from build123d import *

# Parameters (mm, degrees)
F0_W     = 10.922
F0_H     = 25.4
F4_W     = 0.635
F4_H     = 3.81
F6_R     = 1.5875
F7_DEPTH = 12.7
F8_R     = 3.175
F9_DEPTH = 6.35


with BuildPart() as f1:
    # F0 (on Front) → F1 (revolve)
    with BuildSketch(Plane.XZ):
        with Locations((5.461, 0)):
            Rectangle(F0_W, F0_H)
    revolve(axis=Axis((0, 0, 0), (0, 0, -1)))

    # F2 (on face) → F3 (revolve, cut)
    with BuildSketch(Plane(origin=(0, 0, -12.7), x_dir=(1, 0, 0), z_dir=(0, 0, -1))):
        with BuildLine():
            Line((0, 10.287), (0, -10.287))
            ThreePointArc((0, -10.287), (10.287, 0), (0, 10.287))
        make_face()
    revolve(axis=Axis((0, 0, -12.7), (0, 1, 0)), mode=Mode.SUBTRACT)

    # F4 (on Front) → F5 (revolve)
    with BuildSketch(Plane.XZ):
        with Locations((10.6045, -14.605)):
            Rectangle(F4_W, F4_H)
    revolve(axis=Axis((0, 0, -6.3285445794), (0, 0, -1)))

    # F6 (on Right) → F7 (cut, symmetric)
    with BuildSketch(Plane.YZ):
        with Locations((0, -14.478)):
            Circle(F6_R)
    extrude(amount=F7_DEPTH, both=True, mode=Mode.SUBTRACT)

    # F8 (on face) → F9 (join)
    with BuildSketch(Plane.XY.offset(12.7)):
        Circle(F8_R)
    extrude(amount=F9_DEPTH)


solid = f1.part
Build history of the part. All positions in model axes, mm. A direction names the side the tool comes from. Coordinates: 2 decimals unless noted, no trailing zeros. Order: outer loops, then holes, each group sorted by start corner. A loop starts at its lowest first (then second) coordinate and runs counter-clockwise, first axis right, second up. Notation, with made-up numbers: M 34,67 L 89,67 A24 cw 89,82 Z; hole C 23.25,87.5 d11. An arc over 180 degrees is marked long. One line per question, with ' | ' between items. Start each with the question number.
Q1. Saw through at B-B (x = -0.5). List the corners of the cut face in (y, z).
Q2. Saw through at C-C (y = -6.75). List the corners of the cut face in (x, z), then the cut area to 3 significant figures.
Q3. Saw through at D-D (z = -2). List the corners of the cut face in (x, y).
Q4. Saw through at A-A (y = 0). Count the separate pieces of the cut face and the enclosed holes in it, then the cut area to 3 significant figures.
Q5. Flat gauge pins, fed straight in: pin 1 Ø3 at (x, z) = (-3, 9.5) entering from +Y; pin 2 Ø2 at (y, z) = (-2.5, -1.5) entering from -X; pin 3 Ø2 at (x, z) = (1, 4) entering from -Y; pin 4 Ø1.5 at (x, y) = (-0.5, -6.5) entering from -Z. Where does each tip first touch, or does it go through?
Q6. Probe L1, parallel to Z at x = 10.45, y = 0; L2, parallel to Y at x = 0, z = -14.1; L3, parallel to Z at x = -9.5, y = 4.75. List the from-to ranges inside material, lowest first. Write a range as from..to.
Q7. Two-plate mould, pull along Y, no slides. Class faces 3 (the face through (0, 0, 19.05)), 4 (the face through (9.81, -3.09, -14.58)), 5 (the face through (10.09, 4.18, -1.7)): +Y half, -Y half, draft (parallel to the pull), parting line (faces both ways), or undercut.
Q8. 3-axis set-ups, long thin cutter, end or side, ignore diameter. For faces 1 (the face through (-0.69, -3.1, 15.83)), 2 (the face through (10.548, 1.466, -15.086)): which of +Z, -Z, +X, -X, +Y, -Y reach the whole face in a straight line?
Check values:
1) outline: M -10.91,-16.51 L -10.27,-16.51 L -10.27,-12.7 A10.27 cw 10.27,-12.7 L 10.27,-16.51 L 10.91,-16.51 L 10.91,12.7 L 3.14,12.7 L 3.14,19.05 L -3.14,19.05 L -3.14,12.7 L -10.91,12.7 Z
2) outline: M -8.59,-16.51 L -7.76,-16.51 L -7.76,-12.7 A7.76 cw 7.76,-12.7 L 7.76,-16.51 L 8.59,-16.51 L 8.59,12.7 L -8.59,12.7 Z | area: 348 mm2
3) outline: C 0,0 d21.84
4) separate pieces: 3 | enclosed holes: 0 | area: 430 mm2
5) pin 1: stops at y = 10.82 | pin 2: stops at x = -10.82 | pin 3: stops at y = -10.92 | pin 4: stops at z = -5.42
6) L1: z = -16.51..-16.07, -12.89..12.7 | L2: y = -10.92..-10.29, 10.29..10.92 | L3: z = -16.51..12.7
7) face 3: draft | face 4: undercut | face 5: parting line
8) face 1: +Z | face 2: +X, -X
